Work out the finished part from the listing and answer in its coordinate system (mm). Coordinates: 2 decimals unless noted, no trailing zeros. Write each loop counter-clockwise with the first axis right and the second up, starting at its lowest first coordinate (ties: lowest second). Pieces come first, ordered by that corner, then holes. Notation, with made-up numbers: (-22, -27) - (-14, -27) arc R7 cw to (-14, -19) - close; hole circle Ø8 at (-32.75, 85.5). An arc over 180 degrees is marked (long way). Use a Markdown table: item, result. Add a question column.
(1) Given pin 1 Ø1.5 at (x, y) = (2, -12.5) entering from +Z; pin 2 Ø1 at (y, z) = (-1, -1.5) entering from +X; pin 3 Ø9.5 at (x, y) = (-5, -4.5) entering from +Z, each flat-ended and moving along its own axis, determine where each tip first touches the part or whether it passes through.
(2) The part is cut by section A-A, the plane z = -3.5. Give the vertices of the cut face in (x, y), then the cut area to 3 significant figures.
(3) Find the intervals of material crossed by line 1 (Z direction, x = -9.5, y = 5); line 2 (Z direction, x = 9, y = 7); line 3 (X direction, y = 11.5, z = -29), in increasing order. Write a range as from..to.
from build123d import *

# Parameters (mm, degrees)
F0_R     = 10
F1_DEPTH = 20


with BuildPart() as f1:
    # F0 (on Top) → F1 (new body, symmetric)
    with BuildSketch(Plane.XY):
        Circle(F0_R)
    extrude(amount=F1_DEPTH, both=True)

    # F2 (on Right) → F3 (revolve)
    with BuildSketch(Plane.YZ):
        with BuildLine():
            Line((15.806751, -20), (0, -20))
            Line((0, -20), (0, -35.806751))
            ThreePointArc((0, -35.806751), (11.177061, -31.177061), (15.806751, -20))
        make_face()
    revolve(axis=Axis((0, 0, -27.903376), (0, 0, -1)))

    # F4: F1 across plane


with BuildPart() as f1_1:
    add(f1.part)
    add(f1.part.mirror(Plane.XY))


solid = f1_1.part
Model answer:
| question | item | result |
|---|---|---|
| 1 | pin 1 | z = 30.39 |
| 1 | pin 2 | x = 9.99 |
| 1 | pin 3 | z = 35.68 |
| 2 | outline | circle Ø20 at (0, 0) |
| 2 | area | 314 mm^2 |
| 3 | line 1 | -31.6..-20, 20..31.6 |
| 3 | line 2 | -30.95..-20, 20..30.95 |
| 3 | line 3 | -6.05..6.05 |
